from build123d import *

# Parameters (mm, degrees)
ESQUISSE1_R                   = 10
ESQUISSE1_R_2                 = 1.6
BOSS_EXTRU_1_DEPTH            = 2.7
ESQUISSE2_R                   = 4.55
BOSS_EXTRU_2_DEPTH            = 1.9
ESQUISSE5_R                   = 2.75
ENL_V_MAT_EXTRU_1_DEPTH       = 4
DIAM_TRE_DU_PER_AGE_3_0_3_1_D = 3


with BuildPart() as part:
    # Esquisse1 → Boss.-Extru.1 (new body)
    with BuildSketch(Plane(origin=(0, 0, 0), x_dir=(1, 0, 0), z_dir=(0, 1, 0))):
        with Locations(Location((0, 0, 0), (0, 0, 90))):
            Circle(ESQUISSE1_R)
        with Locations(Location((0, 0, 0), (0, 0, 90))):
            Circle(ESQUISSE1_R_2, mode=Mode.SUBTRACT)
    extrude(amount=BOSS_EXTRU_1_DEPTH)

    # Esquisse2 → Boss.-Extru.2 (add)
    with BuildSketch(Plane(origin=(0, 2.7, 0), x_dir=(1, 0, 0), z_dir=(0, 1, 0))):
        with Locations(Location((0, 0, 0), (0, 0, 90))):
            Circle(ESQUISSE2_R)
    extrude(amount=BOSS_EXTRU_2_DEPTH)

    # Esquisse5 → Enlèv. mat.-Extru.1 (cut)
    with BuildSketch(Plane(origin=(0, 4.6, 0), x_dir=(1, 0, 0), z_dir=(0, 1, 0))):
        with Locations(Location((0, 0, 0), (0, 0, 270))):
            Circle(ESQUISSE5_R)
    extrude(amount=-ENL_V_MAT_EXTRU_1_DEPTH, mode=Mode.SUBTRACT)

    # Diamètre du perçage Ø3.0 (3)1 (through all)
    with Locations(Plane(origin=(0, 2.7, 0), x_dir=(1, 0, 0), z_dir=(0, 1, 0))):
        with Locations((4.949747468, -4.949747468), (-4.949747468, -4.949747468), (-4.949747468, 4.949747468), (4.949747468, 4.949747468)):
            Hole(DIAM_TRE_DU_PER_AGE_3_0_3_1_D / 2)


solid = part.part
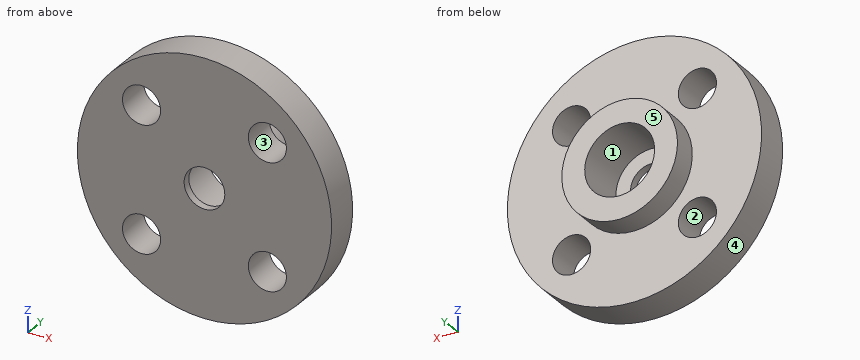
Design review of the part built by this model. Coordinates are the model's own, in mm. Face numbers are marked on the shaded views. A direction names the side the tool comes from. Give positions to 0.01 mm unless a question says otherwise; leave off trailing zeros. Loops run counter-clockwise (first coordinate to the right, second up) from the corner with the lowest first, then second, coordinate; pieces in that order, holes last. Notation, with made-up numbers: M 26.25,9 L 81.25,9 A29 cw 81.25,47 Z; hole C 48,-34 d9. An arc over 180 degrees is marked long. Write item = value, one per line.
Q1. We need section A-A (z = 0). Give the boundary of the cut face in (x, y).
Output values:
outline = M -10,0 L -1.6,0 L -1.6,0.6 L -2.75,0.6 L -2.75,4.6 L -4.55,4.6 L -4.55,2.7 L -10,2.7 Z; M 1.6,0 L 10,0 L 10,2.7 L 4.55,2.7 L 4.55,4.6 L 2.75,4.6 L 2.75,0.6 L 1.6,0.6 Z
Q2. Draft analysis for pull direction X (two halves, no side actions). For the marked faces 3, 4 and 5, state which applies: +X half, -X half, draft (parallel to the pull), parting line (faces both ways), or undercut.
Output values:
face_3 = undercut
face_4 = parting line
face_5 = draft
Q3. We need section D-D (x = 7.5). Give the boundary of the cut face in (y, z).
Output values:
outline = M 0,-6.61 L 2.7,-6.61 L 2.7,6.61 L 0,6.61 Z
Q4. We need section C-C (y = 3.2). Give the boundary of the cut face in (x, z), plus the area to 3 significant figures.
Output values:
outline = C 0,0 d9.1; hole C 0,0 d5.5
area = 41.3 mm^2
Q5. We need section B-B (x = 0). Give the boundary of the cut face in (y, z), plus the area to 3 significant figures.
Output values:
outline = M 0,-10 L 2.7,-10 L 2.7,-4.55 L 4.6,-4.55 L 4.6,-2.75 L 0.6,-2.75 L 0.6,-1.6 L 0,-1.6 Z; M 0,1.6 L 0.6,1.6 L 0.6,2.75 L 4.6,2.75 L 4.6,4.55 L 2.7,4.55 L 2.7,10 L 0,10 Z
area = 47.4 mm^2
Q6. For the marked faces 1 and 2, list the 3-axis set-ups (+Z, -Z, +X, -X, +Y, -Y) from which the entire face can be reached by the end or side of a thin tool; tool diameter is ignored.
Output values:
face_1 = +Y
face_2 = +Y, -Y
Q7. To check wall thickness, follow line 1 (X direction, y = 0.85, z = -5); line 2 (Z direction, x = -6, y = 1.9); line 3 (X direction, y = 2.2, z = 4.5). State the ranges of each line that lie inside material, in increasing order. Write a range as [from, to].
Output values:
line_1 = [-8.66, -6.45], [-3.45, 3.45], [6.45, 8.66]
line_2 = [-8, -6.02], [-3.88, 3.88], [6.02, 8]
line_3 = [-8.93, -6.38], [-3.52, 3.52], [6.38, 8.93]
Q8. Insertion check: pin 1 (3.5 mm diameter, centred on x = 0, z = 0, fed in from +Y); pin 2 (3.5 mm diameter, centred on x = 4.95, z = 4.95, fed in from +Y). Each pin has a flat end and moves straight along its axis. Give the tip position at first contact, or say it passes through.
Output values:
pin_1 = 0.6
pin_2 = 2.7
